Input: part model. Units: mm. Frame: model coordinates. Face numbers are marked on the shaded views. A direction names the side the tool comes from. Give positions to 0.01 mm unless a question says otherwise; leave off trailing zeros. Loops run counter-clockwise (first coordinate to the right, second up) from the corner with the lowest first, then second, coordinate; pieces in that order, holes last. Notation, with made-up numbers: (45, 29) -> (89, 29) arc R26 ccw to (89, 50) -> close; hole circle Ø11 at (-22.5, 18.25). An arc over 180 degrees is marked (long way). Answer as a JSON object with one key per item and string values.
Autodesk Inventor part; units mm, degrees
ref_plane "YZ Plane" through (0, 0, 0) normal (1, 0, 0) x (0, 1, 0)
ref_plane "XZ Plane" through (0, 0, 0) normal (0, 1, 0) x (-1, 0, 0)
ref_plane "XY Plane" through (0, 0, 0) normal (0, 0, 1) x (1, 0, 0)
sketch "Sketch1" plane through (0, 0, 0) normal (0, 1, 0) x (-1, 0, 0)
  circle A0 centre (0, 0) radius 25.4 construction
  line L0 (-28.575, 28.575) -> (28.575, 28.575)
  line L1 (28.575, 28.575) -> (28.575, -28.575)
  line L2 (28.575, -28.575) -> (-28.575, -28.575)
  line L3 (-28.575, -28.575) -> (-28.575, 28.575)
  line L4 (-28.575, 28.575) -> (28.575, -28.575) construction
  line L5 (28.575, 28.575) -> (-28.575, -28.575) construction
  line L6 (26.9875, 26.9875) -> (-26.9875, 26.9875)
  line L7 (-26.9875, 26.9875) -> (-26.9875, -26.9875)
  line L8 (-26.9875, -26.9875) -> (26.9875, -26.9875)
  line L9 (26.9875, -26.9875) -> (26.9875, 26.9875)
  line L10 (26.9875, 26.9875) -> (-26.9875, -26.9875) construction
  line L11 (-26.9875, 26.9875) -> (26.9875, -26.9875) construction
  dimension "d0" = 50.8
  dimension "d1" = 28.575
  dimension "d18" = 53.975
extrude "Extrusion1" add sketch "Sketch1" along normal blind 7.62
extrude "Extrusion2" add sketch "Sketch1" against normal blind 3.175 contours L0 L1 L2 L3 | L9 L8 L7 L6
sketch "Sketch4" plane through (-25.4, -3.175, 28.575) normal (0, 0, 1) x (1, 0, 0)
  line L0 (53.975, 10.795) -> (53.975, 0)
  arc A0 (53.975, 0) -> (-3.175, 0) centre (25.4, -159.4644) ccw
  line L1 (-3.175, 0) -> (53.975, 0) construction
  arc A1 (53.975, -1.5875) -> (-3.175, -1.5875) centre (25.4, -161.0519) ccw
  arc A2 (53.975, -4.7625) -> (-3.175, -4.7625) centre (25.4, -164.2269) ccw
  line L2 (-3.175, -4.7625) -> (-3.175, -1.5875)
  line L3 (-3.175, -1.5875) -> (-3.175, 0)
  line L4 (53.975, -1.5875) -> (53.975, 0)
  line L5 (53.975, -4.7625) -> (53.975, -1.5875)
  point P0 (25.4, 2.54)
  dimension "d56" = 3.175
  dimension "d57" = 1.5875
  dimension "d58" = 2.54
extrude "Extrusion11" add sketch "Sketch4" against normal up to surface (57.15 mm away)
extrude "Extrusion12" cut sketch "Sketch4" against normal blind 44.45 contours L4 A1 L3 A0
extrude "Extrusion13" cut sketch "Sketch4" against normal blind 38.1 contours L5 A2 L2 A1
extrude "Extrusion14" add sketch "Sketch4" against normal blind 12.7 contours L4 A1 L3 A0
extrude "Extrusion15" add sketch "Sketch4" against normal blind 19.05 contours L5 A2 L2 A1
fillet "Fillet6" radius 3.175 4 edges at (28.575, -0.1587, 28.575) (28.575, -0.1587, -28.575) (-28.575, -0.1587, 28.575) (-28.575, -0.1587, -28.575)
sketch "Sketch8" plane through (0, -167.4019, -28.575) normal (0, 0, -1) x (-1, 0, 0)
  line L0 (5, 168.4019) -> (-5, 168.4019)
  line L1 (-5, 168.4019) -> (-5, 167.4019)
  line L2 (-5, 167.4019) -> (6, 167.4019)
  line L3 (-26.9875, 167.4019) -> (26.9875, 167.4019)
  line L4 (6, 167.4019) -> (6, 174.4019)
  line L5 (6, 174.4019) -> (-5, 174.4019)
  line L6 (-5, 174.4019) -> (-5, 173.4019)
  line L7 (-5, 173.4019) -> (5, 173.4019)
  line L8 (5, 173.4019) -> (5, 168.4019)
  line L9 (-5, 173.4019) -> (-5, 168.4019)
  point P0 (0, 167.4019)
  point P1 (0, 168.4019)
  dimension "d68" = 1
  dimension "d74" = 1
  dimension "d75" = 1
  dimension "d76" = 7
  dimension "d77" = 10
extrude "Extrusion16" cut sketch "Sketch8" against normal up to surface (1.5875 mm away) contours L8 L7 L6 L5 L4 L2 L1 L0
extrude "Extrusion17" add sketch "Sketch8" along normal blind 1 contours L0 L9 L7 L8
chamfer "Chamfer3" distance 1 angle 45 4 edges at (0, 6, -29.575) (-5, 3.5, -29.575) (0, 1, -29.575) (5, 3.5, -29.575)
sketch "Sketch9" plane through (-26.9875, 7.62, -26.9875) normal (0, 0, 1) x (1, 0, 0)
  circle A0 centre (26.9875, -4.12) radius 2.5
  line L0 (21.9875, -6.62) -> (21.9875, -1.62)
  point P0 (26.9875, -7.62)
  point P1 (21.9875, -4.12)
  dimension "d83" = 5
extrude "Extrusion18" add sketch "Sketch9" along normal blind 2.6416
properties part number "TrackDisplayBottom"
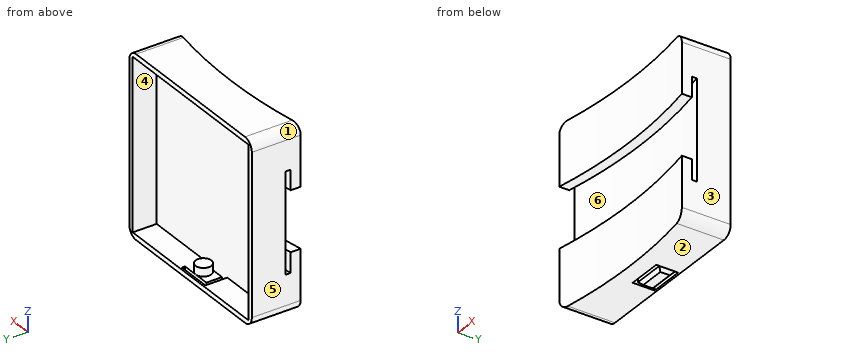
Q1. Draft query along Z for the marked faces 1, 2, 3 and 4. Return one class per face: +Z half, -Z half, draft (parallel to the pull), parting line (faces both ways), or undercut.
Evaluation:
{"face 1": "+Z half", "face 2": "-Z half", "face 3": "draft", "face 4": "undercut"}
Q2. Access query for the marked faces 5 and 6. Directions: +Z, -Z, +X, -X, +Y, -Y. A direction counts if a zero-diameter tool reaches every point of the face in a straight line with its end or side. Return the directions, or none.
Evaluation:
{"face 5": "+Z, -Z, -X, +Y, -Y", "face 6": "none"}
Q3. Section D-D, the plane x = -10. Return the cut outline in (y, z) (1 decimal).
Evaluation:
{"outline": "(-5.7, -28.6) -> (7.6, -28.6) -> (7.6, -27) -> (0, -27) -> (0, 27) -> (7.6, 27) -> (7.6, 28.6) -> (-5.7, 28.6) -> (-5.7, 9.5) -> (-2.5, 9.5) -> (-2.5, 15.9) -> (-0.9, 15.9) -> (-0.9, -15.9) -> (-2.5, -15.9) -> (-2.5, -9.5) -> (-5.7, -9.5) -> close"}
Q4. Section C-C, the plane z = 2.5. Return the cut outline in (x, y) (1 decimal).
Evaluation:
{"outline": "(-28.6, -3.2) arc R162 cw to (28.6, -3.2) -> (28.6, 7.6) -> (27, 7.6) -> (27, 0) -> (-27, 0) -> (-27, 7.6) -> (-28.6, 7.6) -> close"}
Q5. Pin query (flat end, axial travel): pin 1 (0.5 mm diameter, centred on y = 6.5, z = -27.5, fed in from -X); pin 2 (0.8 mm diameter, centred on x = -3, z = -28, fed in from -Y); pin 3 (3 mm diameter, centred on x = -13.5, z = 20, fed in from +Y). Return the tip coordinate at first contact, or that it passes through.
Evaluation:
{"pin 1": "stops at x = -27.98", "pin 2": "stops at y = -5.43", "pin 3": "stops at y = 0"}
Q6. Ray query, line 1 along X through (y, z) = (3.75, 8.5) (1 decimal); line 2 along Z through (x, y) = (-20.5, -4.25) (3 decimals). Return the intervals inside material, ascending.
Evaluation:
{"line 1": "x = -28.6 to -27, 27 to 28.6", "line 2": "z = -28.575 to -9.525, 9.525 to 28.575"}
Q7. Section A-A, the plane z = 13.5. Return the cut outline in (x, y) (1 decimal).
Evaluation:
{"outline": "(-28.6, -7.9) arc R162 cw to (28.6, -7.9) -> (28.6, -4.8) arc R162 ccw to (-28.6, -4.8) -> close; (-28.6, -3.2) arc R162 cw to (28.6, -3.2) -> (28.6, 7.6) -> (27, 7.6) -> (27, 0) -> (-27, 0) -> (-27, 7.6) -> (-28.6, 7.6) -> close"}
